```python
from build123d import *

# Parameters (mm, degrees)
F1_DEPTH = 145
F2_W     = 705
F2_H     = 690
F3_DEPTH = 145.001
F4_W     = 45
F4_H     = 46
F5_DEPTH = 80


with BuildPart() as f1:
    # F0 (on Top) → F1 (new body)
    with BuildSketch(Plane.XY):
        Polygon((397.5, 390), (-397.5, 390), (-397.5, -390), (352.5, -390), (352.5, -435), (397.5, -435), (397.5, -390), align=None)
    extrude(amount=F1_DEPTH)

    # F2 (on face) → F3 (cut, through all)
    with BuildSketch(Plane.XY.offset(145)):
        Rectangle(F2_W, F2_H)
    extrude(amount=-F3_DEPTH, mode=Mode.SUBTRACT)

    # F4 (on face) → F5 (cut)
    with BuildSketch(Plane.XY.offset(145)):
        with Locations((-375, -367)):
            Rectangle(F4_W, F4_H)
    extrude(amount=-F5_DEPTH, mode=Mode.SUBTRACT)


solid = f1.part
```
Verification items for the finished model (mm, model axes). A direction names the side the tool comes from. Coordinates: 2 decimals unless noted, no trailing zeros. Order: outer loops, then holes, each group sorted by start corner. A loop starts at its lowest first (then second) coordinate and runs counter-clockwise, first axis right, second up. Notation, with made-up numbers: (45, 69.5) -> (63, 69.5) arc R13 ccw to (63, 88.5) -> close; hole circle Ø5 at (54, 65). An arc over 180 degrees is marked (long way). Answer as CSV lines item,"result". Start each with the question number.
1) Cross-section at B-B, the plane y = 17. Record the boundary of the cut face in (x, z).
2) Cross-section at A-A, the plane x = 327.5. Record the boundary of the cut face in (y, z), then the cut area to 4 significant figures.
3) Release check for a two-part mould opening along X. For faces 6 (the face through (397.5, -28, 71)), 7 (the face through (-5, -345, 74)), 8 (the face through (-355, 10, 0)) record: released by +X, released by -X, zero draft, split by the parting line, or undercut.
4) Cross-section at D-D, the plane z = 85.5. Record the boundary of the cut face in (x, y).
5) Material ranges on L1, parallel to X at y = -15, z = 134; L2, parallel to Y at x = 91.5, z = 95.5, recorded low to high. Write a range as [from, to].
6) Cross-section at C-C, the plane z = 13. Record the boundary of the cut face in (x, y).
7) Set-up check for faces 1 (the face through (-355, -21, 145)), 2 (the face through (-5, 345, 74)), 3 (the face through (6, 390, 71)), 4 (the face through (-352.5, -368, 106)), 5 (the face through (-28, -390, 71)): record each of +Z, -Z, +X, -X, +Y, -Y from which the full face is reachable in a straight line by a thin tool's end or side.
8) Gauge pin test, flat ends, axial feed: pin 1 Ø22.5 at (x, z) = (-382, 113) entering from -Y; pin 2 Ø13.5 at (y, z) = (-413.5, 82) entering from -X. Record the tip position at first contact, or that the pin passes through.
Conclusion:
1,outline,"(-397.5, 0) -> (-352.5, 0) -> (-352.5, 145) -> (-397.5, 145) -> close; (352.5, 0) -> (397.5, 0) -> (397.5, 145) -> (352.5, 145) -> close"
2,outline,"(-390, 0) -> (-345, 0) -> (-345, 145) -> (-390, 145) -> close; (345, 0) -> (390, 0) -> (390, 145) -> (345, 145) -> close"
2,area,"13,050 mm²"
3,face 6,"released by +X"
3,face 7,"undercut"
3,face 8,"zero draft"
4,outline,"(-397.5, -344) -> (-352.5, -344) -> (-352.5, 345) -> (352.5, 345) -> (352.5, -345) -> (-352.5, -345) -> (-352.5, -390) -> (352.5, -390) -> (352.5, -435) -> (397.5, -435) -> (397.5, 390) -> (-397.5, 390) -> close"
5,L1,"x = [-397.5, -352.5], [352.5, 397.5]"
5,L2,"y = [-390, -345], [345, 390]"
6,outline,"(-397.5, -390) -> (352.5, -390) -> (352.5, -435) -> (397.5, -435) -> (397.5, 390) -> (-397.5, 390) -> close; hole (-352.5, -345) -> (352.5, -345) -> (352.5, 345) -> (-352.5, 345) -> close"
7,face 1,"+Z, +X, -X, +Y, -Y"
7,face 2,"+Z, -Z"
7,face 3,"+Z, -Z, +X, -X, +Y"
7,face 4,"+Z, -X, -Y"
7,face 5,"+Z, -Z, -X, -Y"
8,pin 1,"stops at y = -344"
8,pin 2,"stops at x = 352.5"
